Geometry: see drawing. Coordinates: mm, zero at the bounding-box minimum. A direction names the side the tool comes from. Round coordinates to 2 decimals unless told otherwise and drop trailing zeros. Loops run counter-clockwise (first coordinate to the right, second up) from the corner with the lowest first, then second, coordinate; pieces in that order, holes last.
(1) First-contact query: pin 1 Ø1.6 at (x, y) = (13, 24) entering from -Z; pin 2 Ø10 at (x, z) = (9, 10.5) entering from -Y; pin 3 Ø8 at (x, y) = (6, 16) entering from +Z (3 decimals); pin 4 Ø2 at (x, y) = (21.5, 10.5) entering from -Z. Flat tips, straight axial feed; report the tip coordinate or a pass-through.
(2) Cut plane A-A, the plane y = 12.7. Output: boundary loops of the cut face in (x, z) (1 decimal).
(3) Line query: line 1 (X direction, y = 24.5, z = 8.5) (3 decimals); line 2 (Y direction, x = 2.2, z = 12.7). Output: solid intervals per line, ascending.
(4) Cut plane D-D, the plane x = 24. Output: boundary loops of the cut face in (y, z) (1 decimal), and give its area (3 significant figures).
(5) Cut plane B-B, the plane x = 7.75. Output: boundary loops of the cut face in (y, z) (3 decimals), and give its area (3 significant figures).
(6) Draft query along Y for the marked faces 3, 4 and 5. Return one class per face: released by +Y, released by -Y, zero draft, split by the parting line, or undercut.
(7) Cut plane C-C, the plane z = 79. Output: boundary loops of the cut face in (x, y) (3 decimals).
(8) Access query for the marked faces 1 and 2. Directions: +Z, -Z, +X, -X, +Y, -Y. A direction counts if a zero-diameter tool reaches every point of the face in a straight line with its end or side. Return the directions, or none.
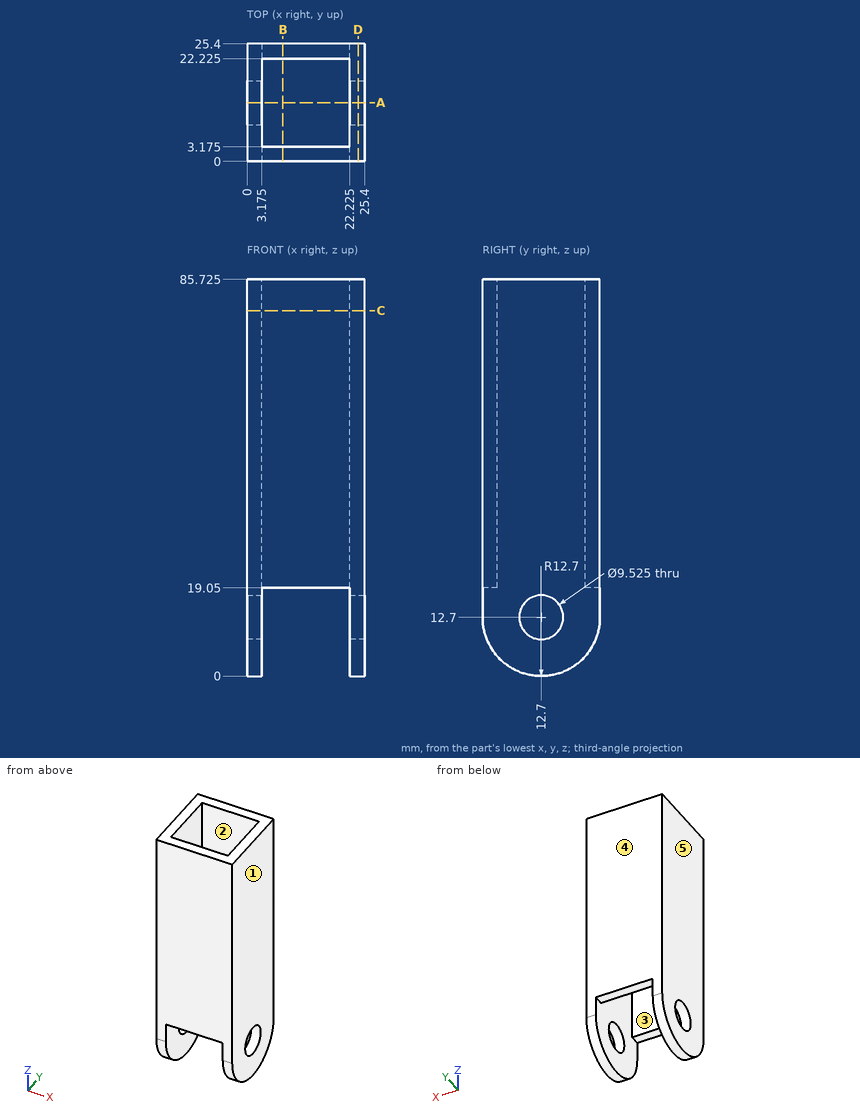
Reported:
1. pin 1: stops at z = 19.05
1. pin 2: passes through
1. pin 3: stops at z = 85.725
1. pin 4: stops at z = 0.09
2. outline: (0, 0) - (3.2, 0) - (3.2, 7.9) - (0, 7.9) - close; (0, 17.5) - (3.2, 17.5) - (3.2, 85.7) - (0, 85.7) - close; (22.2, 0) - (25.4, 0) - (25.4, 7.9) - (22.2, 7.9) - close; (22.2, 17.5) - (25.4, 17.5) - (25.4, 85.7) - (22.2, 85.7) - close
3. line 1: x = 0 to 3.175, 22.225 to 25.4
3. line 2: y = 0 to 7.94, 17.46 to 25.4
4. outline: (0, 12.7) arc R12.7 ccw to (25.4, 12.7) - (25.4, 85.7) - (0, 85.7) - close; hole circle Ø9.5 at (12.7, 12.7)
4. area: 2,040 mm2
5. outline: (0, 19.05) - (3.175, 19.05) - (3.175, 85.725) - (0, 85.725) - close; (22.225, 19.05) - (25.4, 19.05) - (25.4, 85.725) - (22.225, 85.725) - close
5. area: 423 mm2
6. face 3: undercut
6. face 4: released by +Y
6. face 5: zero draft
7. outline: (0, 0) - (25.4, 0) - (25.4, 25.4) - (0, 25.4) - close; hole (3.175, 3.175) - (22.225, 3.175) - (22.225, 22.225) - (3.175, 22.225) - close
8. face 1: +Z, -Z, +X, +Y, -Y
8. face 2: +Z, -Z
